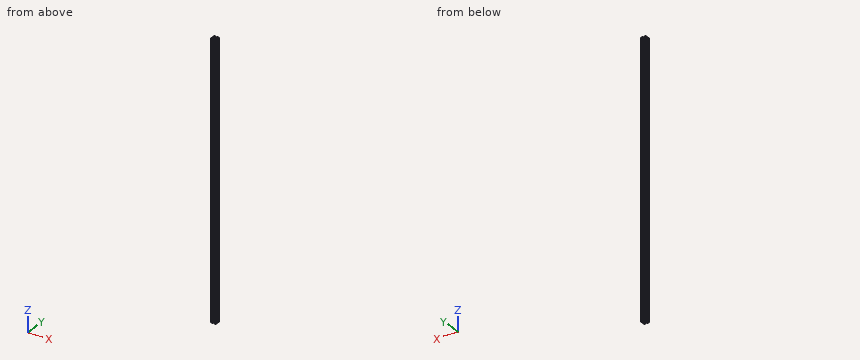
Autodesk Inventor part; units mm, degrees
ref_plane "YZ Plane" through (0, 0, 0) normal (1, 0, 0) x (0, 1, 0)
ref_plane "XZ Plane" through (0, 0, 0) normal (0, 1, 0) x (-1, 0, 0)
ref_plane "XY Plane" through (0, 0, 0) normal (0, 0, 1) x (1, 0, 0)
sketch "Sketch1" plane through (0, 0, 0) normal (0, 0, 1) x (1, 0, 0)
  line L0 (-4.1, -22.5) -> (-4.1, -18)
  line L1 (-4.6, -18) -> (-6.8, -18)
  line L2 (-6.8, -18) -> (-6.8, -9.5)
  line L3 (-6.8, -9.5) -> (-4.5, -7.2)
  line L4 (-4.5, -7.2) -> (4.5, -7.2)
  line L5 (4.5, -7.2) -> (6.8, -9.5)
  line L6 (6.8, -9.5) -> (6.8, -18)
  line L7 (4.1, -18) -> (4.1, -22.5)
  line L8 (22.5, -4.1) -> (18, -4.1)
  line L9 (18, -4.6) -> (18, -6.8)
  line L10 (18, -6.8) -> (9.5, -6.8)
  line L11 (9.5, -6.8) -> (7.2, -4.5)
  line L12 (7.2, -4.5) -> (7.2, 4.5)
  line L13 (7.2, 4.5) -> (9.5, 6.8)
  line L14 (9.5, 6.8) -> (18, 6.8)
  line L15 (18, 4.1) -> (22.5, 4.1)
  line L16 (22.5, 22.5) -> (22.5, 4.4)
  line L17 (4.1, 22.5) -> (4.1, 18)
  line L18 (4.6, 18) -> (6.8, 18)
  line L19 (6.8, 18) -> (6.8, 9.5)
  line L20 (6.8, 9.5) -> (4.5, 7.2)
  line L21 (4.5, 7.2) -> (-4.5, 7.2)
  line L22 (-4.5, 7.2) -> (-6.8, 9.5)
  line L23 (-6.8, 9.5) -> (-6.8, 18)
  line L24 (-4.1, 18) -> (-4.1, 22.5)
  line L25 (-22.5, 22.5) -> (-4.4, 22.5)
  line L26 (-22.5, 4.1) -> (-18, 4.1)
  line L27 (-18, 6.8) -> (-9.5, 6.8)
  line L28 (-9.5, 6.8) -> (-7.2, 4.5)
  line L29 (-7.2, 4.5) -> (-7.2, -4.5)
  line L30 (-7.2, -4.5) -> (-9.5, -6.8)
  line L31 (-9.5, -6.8) -> (-18, -6.8)
  line L32 (-18, -6.8) -> (-18, -4.6)
  line L33 (-18, -4.1) -> (-22.5, -4.1)
  line L34 (-22.5, -22.5) -> (-22.5, -4.4)
  line L35 (-4.4, -22.5) -> (-22.5, -22.5)
  line L36 (-4.5962, -3.182) -> (-3.2627, -1.8485)
  line L37 (-3.2627, 1.8485) -> (-4.5962, 3.182)
  line L38 (-4.5962, 3.182) -> (-3.182, 4.5962)
  line L39 (-3.182, 4.5962) -> (-1.8485, 3.2627)
  line L40 (1.8485, 3.2627) -> (3.182, 4.5962)
  line L41 (3.182, 4.5962) -> (4.5962, 3.182)
  line L42 (4.5962, 3.182) -> (3.2627, 1.8485)
  arc A0 (3.3625, -1.6602) -> (3.3625, 1.6602) centre (0, 0) ccw
  line L43 (3.2627, -1.8485) -> (4.5962, -3.182)
  line L44 (4.5962, -3.182) -> (3.182, -4.5962)
  line L45 (3.182, -4.5962) -> (1.8485, -3.2627)
  line L46 (-1.8485, -3.2627) -> (-3.182, -4.5962)
  line L47 (-3.182, -4.5962) -> (-4.5962, -3.182)
  arc A1 (13.8, -8.8) -> (8.8, -13.8) centre (13.8, -13.8) ccw
  line L48 (13.8, -8.8) -> (20.5, -8.8)
  line L49 (20.5, -8.8) -> (20.5, -15.5)
  arc A2 (15.5, -20.5) -> (20.5, -15.5) centre (15.5, -15.5) ccw
  line L50 (15.5, -20.5) -> (8.8, -20.5)
  line L51 (8.8, -20.5) -> (8.8, -13.8)
  arc A3 (8.8, 13.8) -> (13.8, 8.8) centre (13.8, 13.8) ccw
  line L52 (8.8, 13.8) -> (8.8, 20.5)
  line L53 (8.8, 20.5) -> (15.5, 20.5)
  arc A4 (20.5, 15.5) -> (15.5, 20.5) centre (15.5, 15.5) ccw
  line L54 (20.5, 15.5) -> (20.5, 8.8)
  line L55 (20.5, 8.8) -> (13.8, 8.8)
  arc A5 (-13.8, 8.8) -> (-8.8, 13.8) centre (-13.8, 13.8) ccw
  line L56 (-13.8, 8.8) -> (-20.5, 8.8)
  line L57 (-20.5, 8.8) -> (-20.5, 15.5)
  arc A6 (-15.5, 20.5) -> (-20.5, 15.5) centre (-15.5, 15.5) ccw
  line L58 (-15.5, 20.5) -> (-8.8, 20.5)
  line L59 (-8.8, 20.5) -> (-8.8, 13.8)
  arc A7 (-8.8, -13.8) -> (-13.8, -8.8) centre (-13.8, -13.8) ccw
  line L60 (-8.8, -13.8) -> (-8.8, -20.5)
  line L61 (-8.8, -20.5) -> (-15.5, -20.5)
  arc A8 (-20.5, -15.5) -> (-15.5, -20.5) centre (-15.5, -15.5) ccw
  line L62 (-20.5, -15.5) -> (-20.5, -8.8)
  line L63 (-20.5, -8.8) -> (-13.8, -8.8)
  line L64 (-6.8, 18) -> (-4.1, 18)
  line L65 (4.1, 18) -> (4.6, 18)
  line L66 (-4.4, 22.5) -> (-4.1, 22.5)
  line L67 (4.1, 22.5) -> (22.5, 22.5)
  arc A9 (3.3625, 1.6602) -> (3.2627, 1.8485) centre (0, 0) ccw
  arc A10 (1.8485, 3.2627) -> (-1.6602, 3.3625) centre (0, 0) ccw
  arc A11 (-1.6602, 3.3625) -> (-1.8485, 3.2627) centre (0, 0) ccw
  arc A12 (-3.2627, 1.8485) -> (-3.2627, -1.8485) centre (0, 0) ccw
  arc A13 (-1.8485, -3.2627) -> (-1.6602, -3.3625) centre (0, 0) ccw
  arc A14 (-1.6602, -3.3625) -> (1.8485, -3.2627) centre (0, 0) ccw
  arc A15 (3.2627, -1.8485) -> (3.3625, -1.6602) centre (0, 0) ccw
  line L68 (18, 6.8) -> (18, 4.1)
  line L69 (18, -4.1) -> (18, -4.6)
  line L70 (22.5, 4.4) -> (22.5, 4.1)
  line L71 (22.5, -4.1) -> (22.5, -22.5)
  line L72 (6.8, -18) -> (4.1, -18)
  line L73 (-4.1, -18) -> (-4.6, -18)
  line L74 (22.5, -22.5) -> (4.1, -22.5)
  line L75 (-4.1, -22.5) -> (-4.4, -22.5)
  line L76 (-22.5, -4.4) -> (-22.5, -4.1)
  line L77 (-22.5, 4.1) -> (-22.5, 22.5)
  line L78 (-18, -4.6) -> (-18, -4.1)
  line L79 (-18, 4.1) -> (-18, 6.8)
extrude "Extrusion1" add sketch "Sketch1" along normal blind 2483.024
sketch "Sketch2" plane through (4.1, 22.5, 2483.024) normal (0, 1, 0) x (1, 0, 0)
  line L0 (18.4, 2483.024) -> (18.4, 0)
  line L1 (0, 2483.024) -> (18.4, 2483.024)
  line L2 (9.7, 2483.024) -> (9.7, 0)
  circle A0 centre (9.7, 2467.024) radius 4
  point P0 (-4.1, 2483.024)
  dimension "d2" = 8
  dimension "d3" = 16
  dimension "d4" = 18.4
extrude "Extrusion2" cut sketch "Sketch2" against normal up to next
ref_plane "Work Plane1" through (0, 0, 1241.512) normal (0, 0, -1) x (-1, 0, 0)
mirror "Mirror1" about plane through (0, 0, 1241.512) normal (0, 0, -1) of "Extrusion2"
equation "\"d3\" = 2 * d2"
properties part number "ElectronicCase" material "Aluminum-6061"
CAD build for the part. Positions are in the model's coordinates, mm. Round coordinates to 2 decimals unless told otherwise and drop trailing zeros.
(1) Cut at A-A (z = 1253.5). State how many separate pieces and enclosed holes the cut face has, plus the area to 3 significant figures.
(2) Drop a flat-ended pin along its axis: pin 1 (2 mm diameter, centred on x = -1.5, z = 770, fed in from -Y). Give the stop position or say it passes through.
(3) Wall check: line 1 along X through (y, z) = (-15, 1017); line 2 along X through (y, z) = (-12, 662.5). Give the ranges that are in metal, low to high.
Findings below:
1. separate pieces: 1
1. enclosed holes: 5
1. area: 748 mm2
2. pin 1: stops at y = -7.2
3. line 1: x = -22.5 to -20.5, -8.8 to -6.8, 6.8 to 8.8, 20.5 to 22.5
3. line 2: x = -22.5 to -20.5, -9.14 to -6.8, 6.8 to 9.14, 20.5 to 22.5
